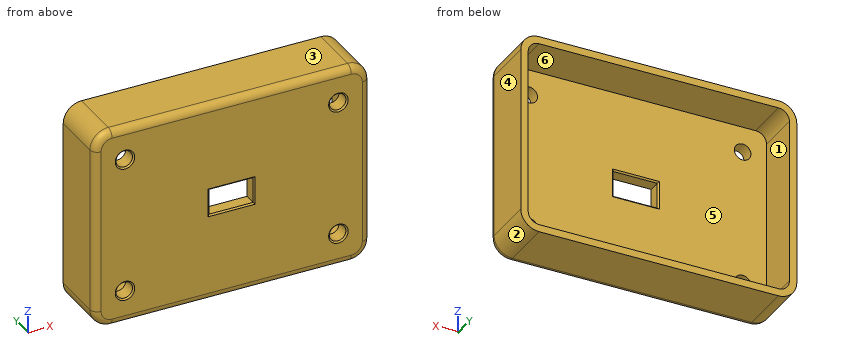
```python
from build123d import *

# Parameters (mm, degrees)
SKETCH1_W           = 75
SKETCH1_H           = 55
BOSS_EXTRUDE1_DEPTH = 4
SKETCH2_W           = 75
SKETCH2_H           = 55
SKETCH2_W_2         = 71
SKETCH2_H_2         = 51
BOSS_EXTRUDE2_DEPTH = 12
SKETCH3_R           = 2.25
SKETCH3_W           = 12
SKETCH3_H           = 7
CUT_EXTRUDE1_DEPTH  = 5
FILLET1_R           = 5
FILLET2_R           = 3
FILLET3_R           = 2
CHAMFER1_SIZE       = 0.4


with BuildPart() as part:
    # Sketch1 → Boss-Extrude1 (new body)
    with BuildSketch(Plane(origin=(0, 0, 0), x_dir=(1, 0, 0), z_dir=(0, 1, 0))):
        Rectangle(SKETCH1_W, SKETCH1_H)
    extrude(amount=BOSS_EXTRUDE1_DEPTH)

    # Sketch2 → Boss-Extrude2 (add)
    with BuildSketch(Plane(origin=(0, 4, 0), x_dir=(1, 0, 0), z_dir=(0, 1, 0))):
        Rectangle(SKETCH2_W, SKETCH2_H)
        Rectangle(SKETCH2_W_2, SKETCH2_H_2, mode=Mode.SUBTRACT)
    extrude(amount=BOSS_EXTRUDE2_DEPTH)

    # Sketch3 → Cut-Extrude1 (cut, through all)
    with BuildSketch(Plane(origin=(0, 4, 0), x_dir=(1, 0, 0), z_dir=(0, 1, 0))):
        with Locations((-29, 18.5)):
            Circle(SKETCH3_R)
        with Locations((29, 18.5)):
            Circle(SKETCH3_R)
        with Locations((29, -18.5)):
            Circle(SKETCH3_R)
        with Locations((-29, -18.5)):
            Circle(SKETCH3_R)
        Rectangle(SKETCH3_W, SKETCH3_H)
    extrude(amount=-CUT_EXTRUDE1_DEPTH, mode=Mode.SUBTRACT)

    # Fillet1
    fillet1_edges = [part.edges().sort_by_distance(p)[0] for p in [
        (37.5, 8, 27.5),
        (-37.5, 8, 27.5),
        (-37.5, 8, -27.5),
        (37.5, 8, -27.5),
    ]]
    fillet(fillet1_edges, radius=FILLET1_R)

    # Fillet2
    fillet2_edges = [part.edges().sort_by_distance(p)[0] for p in [
        (35.5, 10, -25.5),
        (-35.5, 10, -25.5),
        (-35.5, 10, 25.5),
        (35.5, 10, 25.5),
    ]]
    fillet(fillet2_edges, radius=FILLET2_R)

    # Fillet3
    fillet3_edges = [part.edges().sort_by_distance(p)[0] for p in [
        (-37.5, 0, 0),
        (37.5, 0, 0),
        (0, 0, 27.5),
        (0, 0, -27.5),
        (-36.035533906, 0, 26.035533906),
        (36.035533906, 0, 26.035533906),
        (36.035533906, 0, -26.035533906),
        (-36.035533906, 0, -26.035533906),
    ]]
    fillet(fillet3_edges, radius=FILLET3_R)

    # Chamfer1
    chamfer1_edges = [part.edges().sort_by_distance(p)[0] for p in [
        (6, 0, 0),
        (0, 0, 3.5),
        (-6, 0, 0),
        (0, 0, -3.5),
        (6, 4, 0),
        (0, 4, -3.5),
        (-6, 4, 0),
        (0, 4, 3.5),
        (-31.25, 0, 18.5),
        (26.75, 0, 18.5),
        (26.75, 0, -18.5),
        (-31.25, 0, -18.5),
    ]]
    chamfer(chamfer1_edges, length=CHAMFER1_SIZE)


solid = part.part
```
Work out the finished part from the listing and answer in its coordinate system (mm). Face numbers are marked on the shaded views. A direction names the side the tool comes from. Give positions to 0.01 mm unless a question says otherwise; leave off trailing zeros. Order: outer loops, then holes, each group sorted by start corner. A loop starts at its lowest first (then second) coordinate and runs counter-clockwise, first axis right, second up. Notation, with made-up numbers: M 46.25,-29.75 L 97.25,-29.75 A18 cw 97.25,-5.75 Z; hole C 18,56.25 d1. An arc over 180 degrees is marked long. Return JSON: item names as keys, results as strings.
1) Section C-C, the plane x = -3.5 is taken. Write down the section's boundary in (y, z).
Resolved:
{"outline": "M 0,-25.5 A2 ccw 2,-27.5 L 16,-27.5 L 16,-25.5 L 4,-25.5 L 4,-3.9 L 3.6,-3.5 L 0.4,-3.5 L 0,-3.9 Z; M 0,3.9 L 0.4,3.5 L 3.6,3.5 L 4,3.9 L 4,25.5 L 16,25.5 L 16,27.5 L 2,27.5 A2 ccw 0,25.5 Z"}
2) For a pull along Z with two mould halves and no side action, classify the marked faces 3, 4, 5 and 6 as +Z half, -Z half, draft (parallel to the pull), parting line (faces both ways), or undercut.
Resolved:
{"face 3": "+Z half", "face 4": "draft", "face 5": "undercut", "face 6": "undercut"}
3) Section B-B, the plane x = 29 is taken. Write down the section's boundary in (y, z), plus the area to 3 significant figures.
Resolved:
{"outline": "M 0,-25.5 A2 ccw 2,-27.5 L 16,-27.5 L 16,-25.5 L 4,-25.5 L 4,-20.75 L 0.4,-20.75 L 0,-21.15 Z; M 0,-15.85 L 0.4,-16.25 L 4,-16.25 L 4,16.25 L 0.4,16.25 L 0,15.85 Z; M 0,21.15 L 0.4,20.75 L 4,20.75 L 4,25.5 L 16,25.5 L 16,27.5 L 2,27.5 A2 ccw 0,25.5 Z", "area": "230 mm^2"}
4) Section A-A, the plane z = 18.5 is taken. Write down the section's boundary in (x, y), plus the area to 3 significant figures.
Resolved:
{"outline": "M -37.5,2 A2 ccw -35.5,0 L -31.65,0 L -31.25,0.4 L -31.25,4 L -35.5,4 L -35.5,16 L -37.5,16 Z; M -26.75,0.4 L -26.35,0 L 26.35,0 L 26.75,0.4 L 26.75,4 L -26.75,4 Z; M 31.25,0.4 L 31.65,0 L 35.5,0 A2 ccw 37.5,2 L 37.5,16 L 35.5,16 L 35.5,4 L 31.25,4 Z", "area": "310 mm^2"}
5) Straight lines are drawn through the part: line 1 along Z through (x, y) = (-29, 2.15); line 2 along X through (y, z) = (2.35, -18.5); line 3 along X through (y, z) = (4.5, 1). For each, find the intervals that lie inside material, in ascending order. Write a range as [from, to].
Resolved:
{"line 1": "[-27.5, -20.75], [-16.25, 16.25], [20.75, 27.5]", "line 2": "[-37.5, -31.25], [-26.75, 26.75], [31.25, 37.5]", "line 3": "[-37.5, -35.5], [35.5, 37.5]"}
6) A tool of negligible diameter and unlimited length cuts with its end or side. For the marked faces 1 and 2, from which of +Z, -Z, +X, -X, +Y, -Y can it reach the whole face along a straight path? Write none if from no direction.
Resolved:
{"face 1": "+Y", "face 2": "-Z, +X, +Y, -Y"}
7) This flat-tipped pin is pushed along its axis until it touches: pin 1 (6 mm diameter, centred on x = 29, z = 18.5, fed in from +Y). Where does it stop, or does it pass through?
Resolved:
{"pin 1": "y = 4"}
8) Section D-D, the plane y = 10.75 is taken. Write down the section's boundary in (x, z), plus the area to 3 significant figures.
Resolved:
{"outline": "M -37.5,-22.5 A5 ccw -32.5,-27.5 L 32.5,-27.5 A5 ccw 37.5,-22.5 L 37.5,22.5 A5 ccw 32.5,27.5 L -32.5,27.5 A5 ccw -37.5,22.5 Z; hole M -35.5,-22.5 A3 ccw -32.5,-25.5 L 32.5,-25.5 A3 ccw 35.5,-22.5 L 35.5,22.5 A3 ccw 32.5,25.5 L -32.5,25.5 A3 ccw -35.5,22.5 Z", "area": "490 mm^2"}
